from build123d import *

# Parameters (mm, degrees)
BOSS_EXTRUDE1_DEPTH = 2.3
SKETCH7_W           = 2.3
SKETCH7_H           = 10
SKETCH7_W_2         = 10
SKETCH7_H_2         = 2.3
CUT_EXTRUDE2_DEPTH  = 3.3
SKETCH9_R           = 1
CUT_EXTRUDE4_DEPTH  = 3.3
SKETCH10_W          = 3
SKETCH10_H          = 15
SKETCH10_W_2        = 25
SKETCH10_H_2        = 7.5
CUT_EXTRUDE5_DEPTH  = 3.3
FILLET2_R           = 1
FILLET3_R           = 2


with BuildPart() as part:
    # Sketch1 → Boss-Extrude1 (new body)
    with BuildSketch(Plane.XY):
        Polygon((0, -57), (0, -90), (23, -90), (77, -90), (100, -90), (100, -57), (100, 0), (0, 0), align=None)
    extrude(amount=BOSS_EXTRUDE1_DEPTH)

    # Sketch7 → Cut-Extrude2 (cut, through all)
    with BuildSketch(Plane.XY.offset(2.3)):
        with Locations((91, -15)):
            Rectangle(SKETCH7_W, SKETCH7_H)
        with Locations((91, -45)):
            Rectangle(SKETCH7_W, SKETCH7_H)
        with Locations((9, -15)):
            Rectangle(SKETCH7_W, SKETCH7_H)
        with Locations((9, -45)):
            Rectangle(SKETCH7_W, SKETCH7_H)
        with Locations((37.5, -86)):
            Rectangle(SKETCH7_W_2, SKETCH7_H_2)
        with Locations((62.5, -86)):
            Rectangle(SKETCH7_W_2, SKETCH7_H_2)
    extrude(amount=-CUT_EXTRUDE2_DEPTH, mode=Mode.SUBTRACT)

    # Sketch9 → Cut-Extrude4 (cut, through all)
    with BuildSketch(Plane.XY.offset(2.3)):
        with Locations((3, -3)):
            Circle(SKETCH9_R)
        with Locations((97, -3)):
            Circle(SKETCH9_R)
        with Locations((41.13, -11.4)):
            Circle(SKETCH9_R)
        with Locations((69.03, -11.4)):
            Circle(SKETCH9_R)
        with Locations((25.89, -62.2)):
            Circle(SKETCH9_R)
        with Locations((74.11, -63.5)):
            Circle(SKETCH9_R)
    extrude(amount=-CUT_EXTRUDE4_DEPTH, mode=Mode.SUBTRACT)

    # Sketch10 → Cut-Extrude5 (cut, through all)
    with BuildSketch(Plane.XY.offset(2.3)):
        with Locations((17, -22.5)):
            Rectangle(SKETCH10_W, SKETCH10_H)
        with Locations((83, -22.5)):
            Rectangle(SKETCH10_W, SKETCH10_H)
        with Locations((50, -78.75)):
            Rectangle(SKETCH10_W_2, SKETCH10_H_2)
    extrude(amount=-CUT_EXTRUDE5_DEPTH, mode=Mode.SUBTRACT)

    # Fillet2
    fillet2_edges = [part.edges().sort_by_distance(p)[0] for p in [
        (15.5, -30, 1.15),
        (15.5, -15, 1.15),
        (18.5, -15, 1.15),
        (18.5, -30, 1.15),
        (81.5, -30, 1.15),
        (81.5, -15, 1.15),
        (84.5, -15, 1.15),
        (84.5, -30, 1.15),
    ]]
    fillet(fillet2_edges, radius=FILLET2_R)

    # Fillet3
    fillet3_edges = [part.edges().sort_by_distance(p)[0] for p in [
        (37.5, -82.5, 1.15),
        (37.5, -75, 1.15),
        (62.5, -75, 1.15),
        (62.5, -82.5, 1.15),
    ]]
    fillet(fillet3_edges, radius=FILLET3_R)


solid = part.part
Source: CAD feature listing. Evaluate the final solid. Frame: model axes, mm. A direction names the side the tool comes from. Round coordinates to 2 decimals unless told otherwise and drop trailing zeros. Write item = value, one per line. Start each with the question number.
(1) Section query A-A, the plane z = 1.9. State how many separate pieces and enclosed holes the cut face has, plus the area to 3 significant figures.
(2) Pull-direction query (Y, two-part tool) for faces 3 (the face through (49, -44, 0)), 4 (the face through (84.5, -23, 1)); classes: +Y half, -Y half, draft (parallel to the pull), parting line (faces both ways), or undercut.
(3) Set-up query: faces 1 (the face through (9, -40, 1)), 2 (the face through (0, -44, 1)). Return all of +Z, -Z, +X, -X, +Y, -Y with unobstructed straight access to the full face (end or side cutting, diameter ignored); none if empty.
(4) Pin query (flat end, axial travel): pin 1 (1.5 mm diameter, centred on x = 28.5, y = -31.5, fed in from -Z); pin 2 (1.6 mm diameter, centred on x = 3, y = -3, fed in from +Z). Return the tip coordinate at first contact, or that it passes through.
(5) Ray query, line 1 along Y through (x, z) = (90, 1.25); line 2 along X through (y, z) = (-17, 1.5); line 3 along X through (y, z) = (-48.5, 1.85). Return the intervals inside material, ascending. Write a range as from..to.
Conclusion:
q1.separate_pieces = 1
q1.enclosed_holes = 15
q1.area = 8,570 mm2
q2.face_3 = draft
q2.face_4 = undercut
q3.face_1 = +Z, -Z
q3.face_2 = +Z, -Z, -X, +Y, -Y
q4.pin_1 = 0
q4.pin_2 = through
q5.line_1 = -90..-50, -40..-20, -10..0
q5.line_2 = 0..7.85, 10.15..15.5, 18.5..81.5, 84.5..89.85, 92.15..100
q5.line_3 = 0..7.85, 10.15..89.85, 92.15..100
